The drawing under review shows one solid part. Ordinate dimensions are in mm from its lowest x, y, z. A direction names the side the tool comes from. Coordinates: 2 decimals unless noted, no trailing zeros. Order: outer loops, then holes, each group sorted by start corner. A loop starts at its lowest first (then second) coordinate and runs counter-clockwise, first axis right, second up. Notation, with made-up numbers: M -13.5,-38 L 13.5,-38 A21 ccw 13.5,-25 Z; hole C 33,-5.75 d5. An arc over 180 degrees is marked long. Answer as a JSON object with one key per item and string values.
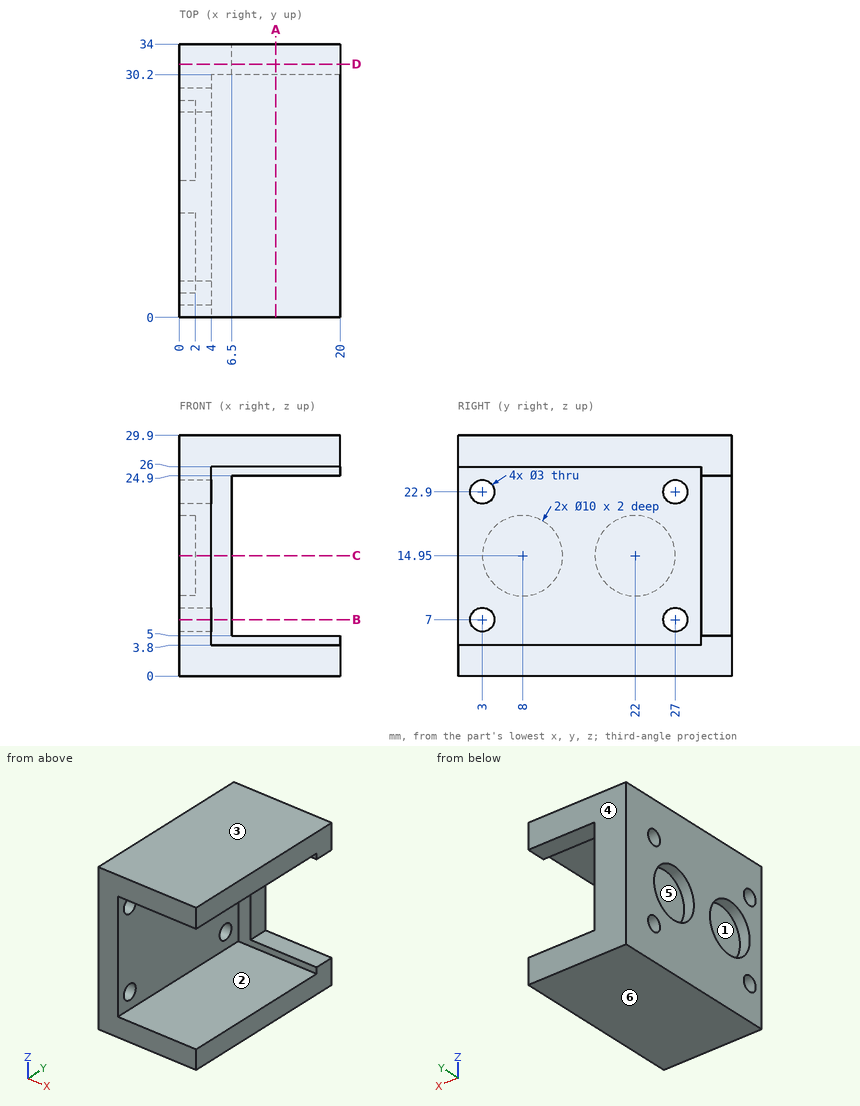
1) Insertion check: pin 1 Ø1.5 at (y, z) = (23, 4.5) entering from -X; pin 2 Ø11.5 at (y, z) = (22, 14.95) entering from +X; pin 3 Ø4 at (y, z) = (32, 19) entering from +X; pin 4 Ø9 at (y, z) = (8, 14.95) entering from -X. Each pin has a flat end and moves straight along its axis. Give the tip position at first contact, or say it passes through.
Taken from the geometry:
{"pin 1": "stops at x = 0", "pin 2": "stops at x = 4", "pin 3": "stops at x = 6.5", "pin 4": "stops at x = 2"}
2) Add section A-A (x = 12). State the section outline as (y, z) points, and give its area (3 significant figures).
Taken from the geometry:
{"outline": "M 0,0 L 34,0 L 34,5 L 30.2,5 L 30.2,3.8 L 0,3.8 Z; M 0,26 L 30.2,26 L 30.2,24.9 L 34,24.9 L 34,29.9 L 0,29.9 Z", "area": "271 mm2"}
3) Add section C-C (z = 14.95). State the section outline as (x, y) points, and give its area (4 significant figures).
Taken from the geometry:
{"outline": "M 0,0 L 4,0 L 4,30.2 L 6.5,30.2 L 6.5,34 L 0,34 L 0,27 L 2,27 L 2,17 L 0,17 L 0,13 L 2,13 L 2,3 L 0,3 Z", "area": "105.5 mm2"}
4) Mouldability with a two-part tool opening along Y and no side actions: class the marked faces 4, 5 and 6 as released by +Y, released by -Y, zero draft, split by the parting line, or undercut.
Taken from the geometry:
{"face 4": "released by +Y", "face 5": "undercut", "face 6": "zero draft"}
5) Tool access review of the marked faces 1, 2 and 3: name each direction out of +Z, -Z, +X, -X, +Y, -Y from which nothing blocks a thin tool from reaching the whole face with its end or side.
Taken from the geometry:
{"face 1": "-X", "face 2": "+X, -Y", "face 3": "+Z, +X, -X, +Y, -Y"}
6) To check wall thickness, follow L1, parallel to Y at x = 1.8, z = 7; L2, parallel to Z at x = 9, y = 11.5; L3, parallel to Z at x = 13.25, y = 30.5. State the ranges of each line that lie inside material, in increasing order.
Taken from the geometry:
{"L1": "y = 0 to 1.5, 4.5 to 25.5, 28.5 to 34", "L2": "z = 0 to 3.8, 26 to 29.9", "L3": "z = 0 to 5, 24.9 to 29.9"}
7) Add section B-B (z = 7). State the section outline as (x, y) points, and give its area (4 significant figures).
Taken from the geometry:
{"outline": "M 0,0 L 4,0 L 4,1.5 L 0,1.5 Z; M 0,4.5 L 4,4.5 L 4,25.5 L 0,25.5 Z; M 0,28.5 L 4,28.5 L 4,30.2 L 6.5,30.2 L 6.5,34 L 0,34 Z", "area": "121.5 mm2"}
8) Add section D-D (y = 31.5). State the section outline as (x, z) points.
Taken from the geometry:
{"outline": "M 0,0 L 20,0 L 20,5 L 6.5,5 L 6.5,24.9 L 20,24.9 L 20,29.9 L 0,29.9 Z"}
